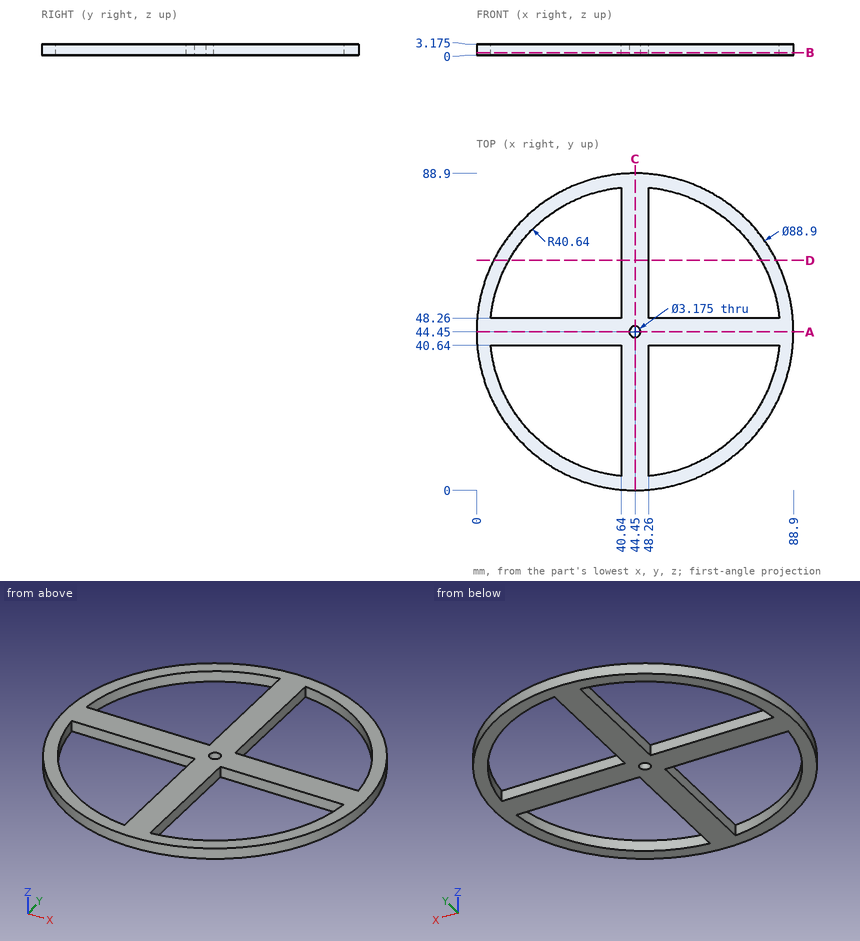
Input: dimensioned drawing with shaded views. Units: mm. Origin: part minimum x, y, z. Give positions to 0.01 mm unless a question says otherwise; leave off trailing zeros. Order: outer loops, then holes, each group sorted by start corner. A loop starts at its lowest first (then second) coordinate and runs counter-clockwise, first axis right, second up.
(1) Material intervals for line 1 along X through (y, z) = (56, 2.3); line 2 along Y through (x, z) = (67.5, 2.85); line 3 along Y through (x, z) = (44.45, 0.7), sorted ascending.
(2) Section query D-D (y = 64.5). Return the cut outline in (x, z) (3 decimals), plus the area to 3 significant figures.
(3) Section query A-A (y = 44.45). Return the cut outline in (x, z) (1 decimal), plus the area to 3 significant figures.
(4) Contact query for flat-ended pins moving along their axis: P1, Ø1, axis at y = 75, z = 1.5, coming from the -X side; P2, Ø1.5, axis at y = 25, z = 3, coming from the +X side; P3, Ø1.6, axis at y = 24, z = 2.5, coming from the -X side. Output: stop coordinate, or through.
(5) Section query B-B (z = 0.75). State how many separate pieces and enclosed holes the cut face has, plus the area to 3 significant figures.
Outcome:
1. line 1: x = 1.53 to 5.49, 40.64 to 48.26, 83.41 to 87.37
1. line 2: y = 6.44 to 10.98, 40.64 to 48.26, 77.92 to 82.46
1. line 3: y = 0 to 42.86, 46.04 to 88.9
2. outline: (4.779, 0) - (9.1, 0) - (9.1, 3.175) - (4.779, 3.175) - close; (40.64, 0) - (48.26, 0) - (48.26, 3.175) - (40.64, 3.175) - close; (79.8, 0) - (84.121, 0) - (84.121, 3.175) - (79.8, 3.175) - close
2. area: 51.6 mm2
3. outline: (0, 0) - (42.9, 0) - (42.9, 3.2) - (0, 3.2) - close; (46, 0) - (88.9, 0) - (88.9, 3.2) - (46, 3.2) - close
3. area: 272 mm2
4. P1: stops at x = 11.7
4. P2: stops at x = 84.78
4. P3: stops at x = 4.58
5. separate pieces: 1
5. enclosed holes: 5
5. area: 2,190 mm2
